Verification items for this drawing (mm, ordinates from the low corner). Round coordinates to 2 decimals unless told otherwise and drop trailing zeros. Loops run counter-clockwise (first coordinate to the right, second up) from the corner with the lowest first, then second, coordinate; pieces in that order, holes last. Notation, with made-up numbers: (79.5, -23.75) - (110.5, -23.75) arc R23 ccw to (110.5, -6.75) - close; hole circle Ø4 at (-13.5, 68.5). An arc over 180 degrees is marked (long way). Put each result on its own line as item: value. Start each with the question number.
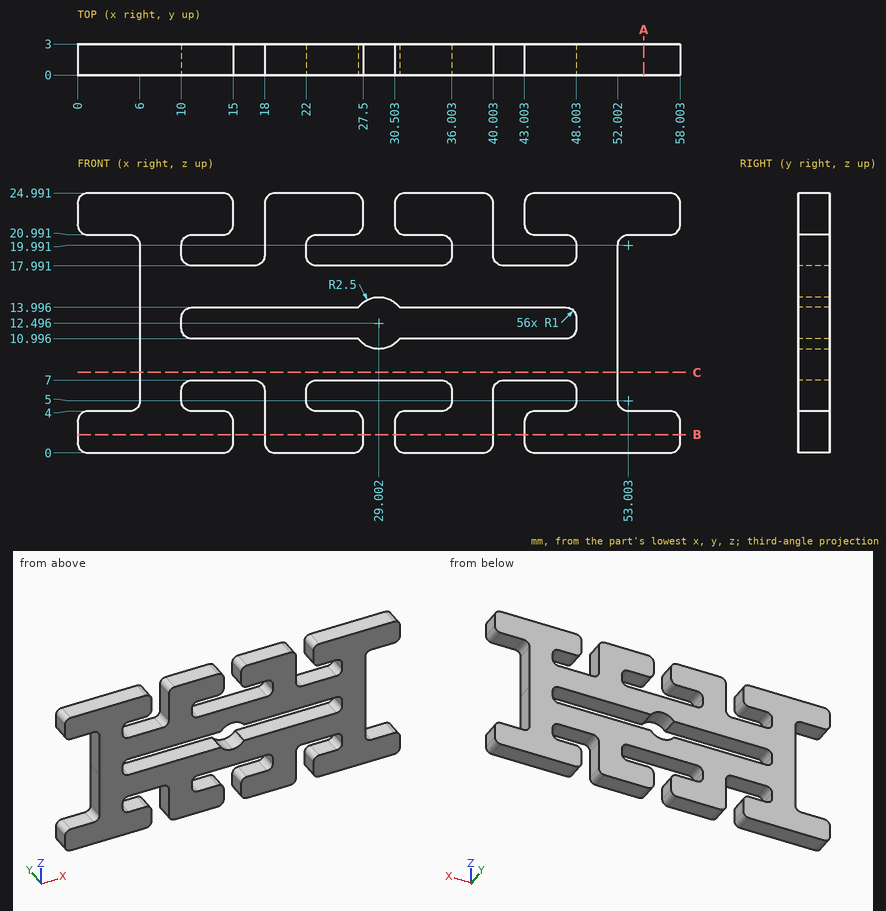
Q1. Cross-section at A-A on x = 54.5. Enter the section's corners in (y, z).
Q2. Cross-section at B-B on z = 1.75. Enter the section's corners in (x, y), and give its area (3 significant figures).
Q3. Cross-section at C-C on z = 7.75. Enter the section's corners in (x, y).
Q4. Depth check by flat-ended pin: pin 1 Ø1.5 at (x, z) = (45.5, 19.5) entering from -Y; pin 2 Ø1.1 at (y, z) = (1.5, 5.5) entering from -X; pin 3 Ø0.5 at (y, z) = (1, 12.5) entering from +X. Enter the tip coordinate at first touch or a pass-through.
Q5. Material ranges on line 1 (X direction, y = 0.4, z = 22); line 2 (X direction, y = 0.35, z = 20); line 3 (Z direction, x = 12, y = 1.7) (1 decimal), recorded low to high. Write a range as from..to.
Answer list:
1. outline: (0, 0) - (3, 0) - (3, 4) - (0, 4) - close; (0, 20.99) - (3, 20.99) - (3, 24.99) - (0, 24.99) - close
2. outline: (0, 0) - (15, 0) - (15, 3) - (0, 3) - close; (18, 0) - (27.5, 0) - (27.5, 3) - (18, 3) - close; (30.5, 0) - (40, 0) - (40, 3) - (30.5, 3) - close; (43, 0) - (58, 0) - (58, 3) - (43, 3) - close
2. area: 147 mm2
3. outline: (6, 0) - (52, 0) - (52, 3) - (6, 3) - close
4. pin 1: passes through
4. pin 2: stops at x = 6
4. pin 3: stops at x = 52
5. line 1: x = 0..15, 18..27.5, 30.5..40, 43..58
5. line 2: x = 6..10, 18..22, 36..40, 48..52
5. line 3: z = 0..4, 7..11, 14..18, 21..25
